Source: three-view drawing plus pictorial views. Frame: mm from the lowest corner of the part. A direction names the side the tool comes from. Give positions to 0.01 mm unless a question says otherwise; leave off trailing zeros. Order: outer loops, then holes, each group sorted by start corner. A loop starts at its lowest first (then second) coordinate and runs counter-clockwise, first axis right, second up.
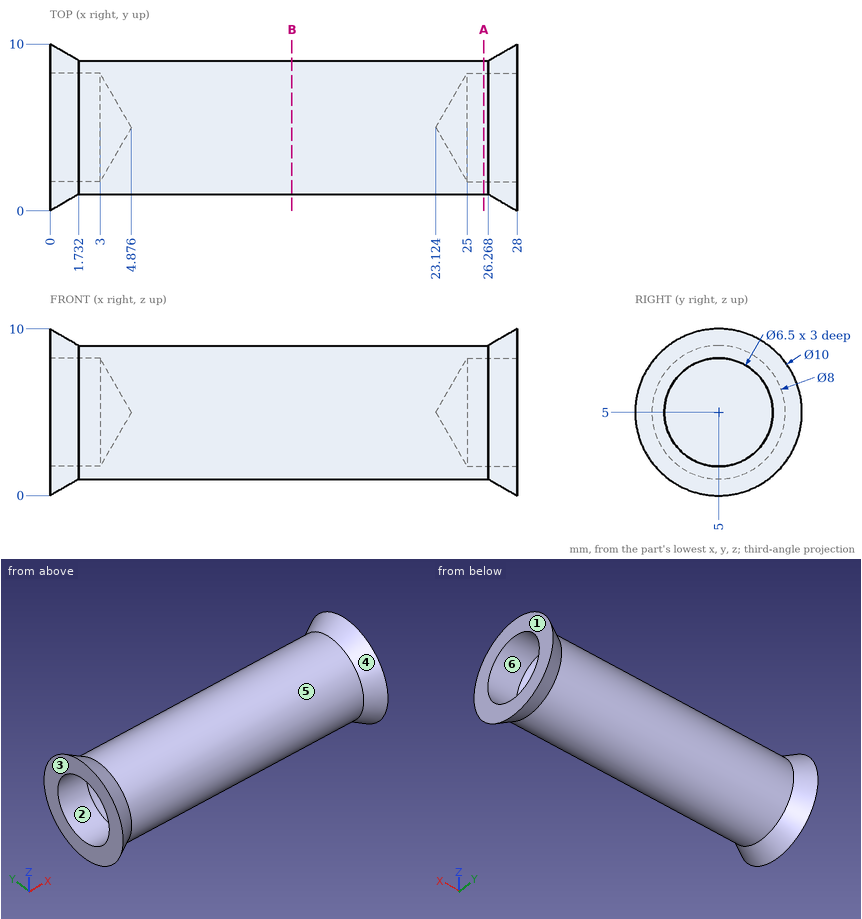
(1) Draft query along X for the marked faces 1, 2, 3 and 4. Return one class per face: +X half, -X half, draft (parallel to the pull), parting line (faces both ways), or undercut.
(2) Pin query (flat end, axial travel): pin 1 Ø1.5 at (y, z) = (7, 5.5) entering from +X; pin 2 Ø1 at (x, z) = (23.5, 8.5) entering from +Y (1 decimal); pin 3 Ø6 at (x, y) = (21.5, 8) entering from -Z. Return the tip coordinate at first contact, or that it passes through.
(3) Access query for the marked faces 5 and 6. Directions: +Z, -Z, +X, -X, +Y, -Y. A direction counts if a zero-diameter tool reaches every point of the face in a straight line with its end or side. Return the directions, or none.
(4) Line query: line 1 along Z through (x, y) = (1.75, 5); line 2 along Y through (x, z) = (0.8, 5); line 3 along Z through (x, y) = (2.25, 3) (1 decimal). Output: solid intervals per line, ascending.
(5) Section B-B, the plane x = 14.5. Return loops of the section in (y, z).
(6) Section A-A, the plane x = 26. Return loops of the section in (y, z).
Checks:
1. face 1: +X half
1. face 2: draft
1. face 3: -X half
1. face 4: undercut
2. pin 1: stops at x = 24.75
2. pin 2: stops at y = 7.6
2. pin 3: stops at z = 1
3. face 5: none
3. face 6: +X
4. line 1: z = 1 to 1.75, 8.25 to 9
4. line 2: y = 0.46 to 1.75, 8.25 to 9.54
4. line 3: z = 1.5 to 2.4, 7.6 to 8.5
5. outline: circle Ø8 at (5, 5)
6. outline: circle Ø8 at (5, 5); hole circle Ø6.5 at (5, 5)
